Build history of the part. All positions in model axes, mm. Face numbers are marked on the shaded views. A direction names the side the tool comes from. Round coordinates to 2 decimals unless told otherwise and drop trailing zeros. Loops run counter-clockwise (first coordinate to the right, second up) from the corner with the lowest first, then second, coordinate; pieces in that order, holes last. Notation, with made-up numbers: (74, -36.5) - (85, -36.5) arc R10 cw to (85, -27.5) - close; hole circle Ø9 at (-39, 49). An arc over 180 degrees is marked (long way). Use one line per item in the form item = value. Start each with the question number.
Q1. Saw through at D-D (z = 6.5). Give the cut face in (x, y), then the cut area to 3 significant figures.
Q2. Saw through at A-A (z = 0.5). Give the cut face in (x, y), then the cut area to 3 significant figures.
Q3. Saw through at B-B (x = 5). Give the cut face in (y, z), then the cut area to 3 significant figures.
Q4. Saw through at C-C (y = 6.75). Give the cut face in (x, z), then the cut area to 3 significant figures.
Q5. Drill centre lines: line 1 (Z direction, x = 10, y = 9.5); line 2 (Z direction, x = 9, y = 7.25); line 3 (Y direction, x = 6.5, z = 5.5). Where is each one in solid material? Low to high.
Q6. Pin check, flat tips, straight feed: pin 1 (5 mm diameter, centred on x = 6.5, z = 5.5, fed in from +Y); pin 2 (5.5 mm diameter, centred on x = 6, y = 18, fed in from +Z); pin 3 (5.5 mm diameter, centred on x = 9, z = 5, fed in from +Y). Stop position of each tip, or through.
Q7. 3-axis set-ups, long thin cutter, end or side, ignore diameter. For the marked faces 1 and 2: which of +Z, -Z, +X, -X, +Y, -Y reach the whole face in a straight line?
```python
from build123d import *

# Parameters (mm, degrees)
EXTRUDE_1_DEPTH = 5
EXTRUDE_2_DEPTH = 10
EXTRUDE_4_DEPTH = 20
EXTRUDE_5_DEPTH = 15


with BuildPart() as part:
    # Sketch 1 → Extrude 1 (new body)
    with BuildSketch(Plane(origin=(0, 0, 0), x_dir=(1, 0, 0), z_dir=(0, 1, 0))):
        Polygon((12.5, -10), (12.5, 0), (7.5, -10), align=None)
        Polygon((12.5, 0), (7.5, 0), (2.5, -10), (7.5, -10), align=None)
        Polygon((7.5, 0), (2.5, 0), (-2.5, -10), (2.5, -10), align=None)
        Polygon((-2.5, -10), (2.5, 0), (7.5, 0), (12.5, 10), (-12.5, 10), (-12.5, -10), align=None)
        Polygon((12.5, 10), (7.5, 0), (12.5, 0), align=None)
    extrude(amount=EXTRUDE_1_DEPTH)

    # Sketch 1_3 → Extrude 2 (add)
    with BuildSketch(Plane(origin=(0, 0, 0), x_dir=(1, 0, 0), z_dir=(0, 1, 0))):
        Polygon((12.5, 0), (7.5, 0), (2.5, -10), (7.5, -10), align=None)
        Polygon((12.5, 10), (7.5, 0), (12.5, 0), align=None)
        Polygon((7.5, 0), (2.5, 0), (-2.5, -10), (2.5, -10), align=None)
        Polygon((-2.5, -10), (2.5, 0), (7.5, 0), (12.5, 10), (-12.5, 10), (-12.5, -10), align=None)
    extrude(amount=EXTRUDE_2_DEPTH)

    # Sketch 1_5 → Extrude 4 (add)
    with BuildSketch(Plane(origin=(0, 0, 0), x_dir=(1, 0, 0), z_dir=(0, 1, 0))):
        Polygon((-2.5, -10), (2.5, 0), (7.5, 0), (12.5, 10), (-12.5, 10), (-12.5, -10), align=None)
    extrude(amount=EXTRUDE_4_DEPTH)

    # Sketch 1_6 → Extrude 5 (add)
    with BuildSketch(Plane(origin=(0, 0, 0), x_dir=(1, 0, 0), z_dir=(0, 1, 0))):
        Polygon((12.5, 10), (7.5, 0), (12.5, 0), align=None)
        Polygon((7.5, 0), (2.5, 0), (-2.5, -10), (2.5, -10), align=None)
    extrude(amount=EXTRUDE_5_DEPTH)


solid = part.part
```
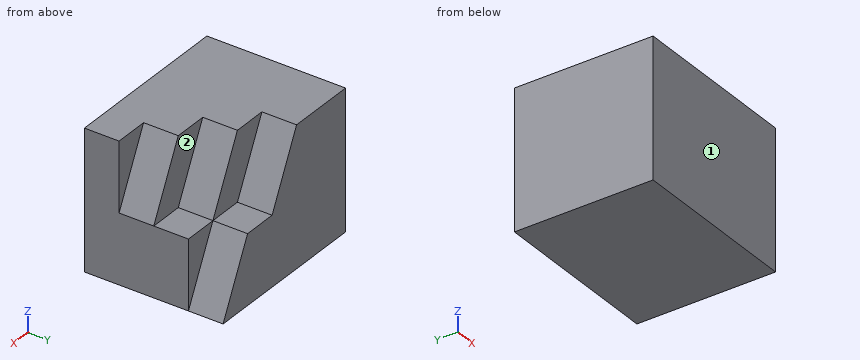
Report:
q1.outline = (-12.5, 0) - (12.5, 0) - (12.5, 5) - (9.25, 5) - (9.25, 10) - (4.25, 10) - (4.25, 15) - (-0.75, 15) - (-0.75, 20) - (-12.5, 20) - close
q1.area = 376 mm²
q2.outline = (-12.5, 0) - (12.5, 0) - (12.5, 5) - (12.25, 5) - (12.25, 10) - (7.25, 10) - (7.25, 15) - (2.25, 15) - (2.25, 20) - (-12.5, 20) - close
q2.area = 421 mm²
q3.outline = (0, -10) - (20, -10) - (20, 0) - (15, 0) - (15, 5) - (10, 5) - (10, 10) - (0, 10) - close
q3.area = 325 mm²
q4.outline = (-12.5, -10) - (12.5, -10) - (12.5, 0) - (7.5, 10) - (-12.5, 10) - close
q4.area = 475 mm²
q5.line_1 = -10 to 5
q5.line_2 = -10 to 7
q5.line_3 = 0 to 10
q6.pin_1 = 15
q6.pin_2 = 0
q6.pin_3 = 10
q7.face_1 = +Z, -Z, +X, -X, -Y
q7.face_2 = +Z, +X, +Y
